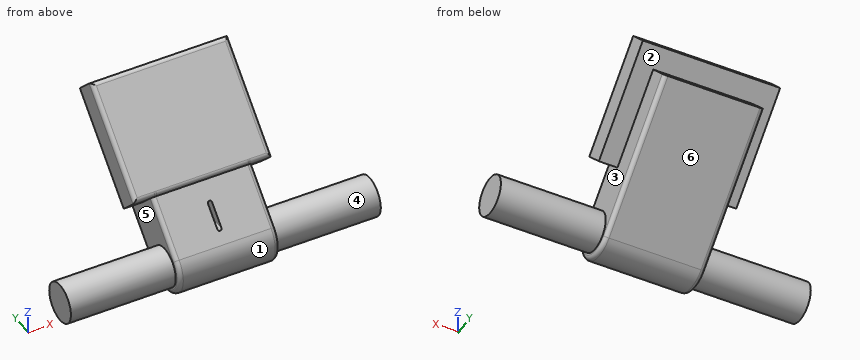
```python
from build123d import *

# Parameters (mm, degrees)
F3_DEPTH  = 61.595
F4_W      = 168.91
F4_H      = 138.43
F5_DEPTH  = 34.29
F6_W      = 80.128736575
F6_H      = 24.2466915269
F7_DEPTH  = 2.54
F8_R      = 1.778
F9_R      = 5.08
F10_R     = 5.08
F11_R     = 24.13
F12_DEPTH = 190.5


with BuildPart() as f3:
    # F2 (on Right) → F3 (new body, symmetric)
    with BuildSketch(Plane.YZ):
        with BuildLine():
            Line((29.2756349547, 74.17691556), (-22.4506403027, 22.4506403027))
            ThreePointArc((-22.4506403027, 22.4506403027), (-22.4506403027, -22.4506403027), (22.4506403027, -22.4506403027))
            Line((22.4506403027, -22.4506403027), (153.7419847927, 108.8407041874))
            Line((153.7419847927, 108.8407041874), (129.8545035107, 132.7281854694))
            Line((129.8545035107, 132.7281854694), (50.289434278, 53.1631162367))
            Line((50.289434278, 53.1631162367), (29.2756349547, 74.17691556))
        make_face()
    extrude(amount=F3_DEPTH, both=True)

    # F4 (on face) → F5 (join)
    with BuildSketch(Plane(origin=(0, -1.4368409794, 1.4368409794), x_dir=(1, 0, 0), z_dir=(0, -0.7071067812, 0.7071067812))):
        with Locations((0, 142.367)):
            Rectangle(F4_W, F4_H)
    extrude(amount=F5_DEPTH)

    # F6 (on Right) → F7 (cut, symmetric)
    with BuildSketch(Plane.YZ):
        with Locations((-11.494727835, 45.5298985338)):
            Rectangle(F6_W, F6_H)
    extrude(amount=F7_DEPTH, both=True, mode=Mode.SUBTRACT)

    # F8
    f8_edges = [f3.edges().sort_by_distance(p)[0] for p in [
        (2.54, 20.660802, 57.653244),
        (-2.54, 20.660802, 57.653244),
        (2.54, 8.537456, 33.406553),
        (-2.54, 8.537456, 33.406553),
    ]]
    fillet(f8_edges, radius=F8_R)

    # F9
    f9_edges = [f3.edges().sort_by_distance(p)[0] for p in [
        (-61.595, 3.412497, 48.313778),
        (61.595, 3.412497, 48.313778),
    ]]
    fillet(f9_edges, radius=F9_R)

    # F10
    f10_edges = [f3.edges().sort_by_distance(p)[0] for p in [
        (84.455, 74.985139, 126.352204),
        (0, 123.927534, 175.294599),
        (-84.455, 74.985139, 126.352204),
        (0, 26.042743, 77.409808),
    ]]
    fillet(f10_edges, radius=F10_R)

    # F11 (on Right) → F12 (join, symmetric)
    with BuildSketch(Plane.YZ):
        Circle(F11_R)
    extrude(amount=F12_DEPTH, both=True)


solid = f3.part
```
Model file for the job. Use its own axes, mm. Face numbers are marked on the shaded views. A direction names the side the tool comes from. Round coordinates to 2 decimals unless told otherwise and drop trailing zeros. Write each loop counter-clockwise with the first axis right and the second up, starting at its lowest first coordinate (ties: lowest second). Pieces come first, ordered by that corner, then holes. Notation, with made-up numbers: M 86,66.25 L 107,66.25 A25 cw 107,88.25 Z; hole C 39.5,81.5 d3. An arc over 180 degrees is marked long. Put each result on its own line as item: value.
Item 1: Flat gauge pins, fed straight in: P1, Ø1.5, axis at y = 68.5, z = 85.5, coming from the +X side (3 decimals); P2, Ø5, axis at y = 42.5, z = 16.5, coming from the -X side (3 decimals); P3, Ø6, axis at x = 102, y = -2, coming from the -Z side. Where does each tip first touch, or does it go through?
Responses:
P1: x = 84.455
P2: x = -61.595
P3: z = -24.13
Item 2: Cut at A-A (x = 138). List the corners of the cut face in (y, z).
Responses:
outline: C 0,0 d48.26
Item 3: Probe L1, parallel to X at y = 93.5, z = 86 (3 decimals); L2, parallel to Y at x = 35.5, z = 67; L3, parallel to Y at x = -19.5, z = 40. List the from-to ranges inside material, lowest first. Write a range as from..to.
Responses:
L1: -61.595..61.595
L2: 22.1..111.9
L3: -4.9..84.9
Item 4: Tool access for the marked faces 4, 5 and 6: list every direction of +Z, -Z, +X, -X, +Y, -Y with a clear straight run to the whole face (end or side of a thin tool).
Responses:
face 4: +X
face 5: -X
face 6: -Z, +X, -X, +Y
Item 5: Mould opens along Z. For the marked faces 1, 2 and 3 say: +Z half, -Z half, draft (parallel to the pull), parting line (faces both ways), or undercut.
Responses:
face 1: parting line
face 2: undercut
face 3: draft
